Part model, mm, in its own coordinate system. Round coordinates to 2 decimals unless told otherwise and drop trailing zeros.
1) Mould opens along Y. For faces 1 (the flat face through (23132, 25, 11389)), 2 (the flat face through (23132, 0, 11389)) say: +Y half, -Y half, draft (parallel to the pull), parting line (faces both ways), or undercut.
2) Probe line 1 (Z direction, x = 23133, y = 11); line 2 (Z direction, x = 23136, y = 1.5); line 3 (X direction, y = 19.25, z = 10180.5). List the from-to ranges inside material, lowest first.
3) Drop a flat-ended pin along its axis: P1, Ø3, axis at x = 23140.5, z = 10486.5, coming from the -Y side. Give the stop position or say it passes through.
from build123d import *

# Parameters (mm, degrees)
SKETCH4_W             = 200
SKETCH4_H             = 2933.573874127
SKETCH4_R             = 12.5
BOSS_EXTRUDE1_DEPTH   = 25
SKETCH4_H_2           = 2891.000919938
BOSS_EXTRUDE1_2_DEPTH = 25
SKETCH4_H_3           = 2656.8496719
BOSS_EXTRUDE1_3_DEPTH = 25
SKETCH4_H_4           = 2167.26069873
BOSS_EXTRUDE1_4_DEPTH = 25
SKETCH4_H_5           = 1693.636583381
BOSS_EXTRUDE1_5_DEPTH = 25
SKETCH5_W             = 5252.2870397
SKETCH5_H             = 5093.660921052
CUT_EXTRUDE3_DEPTH    = 26


with BuildPart() as part:
    # Sketch4 → Boss-Extrude1 (new body)
    with BuildSketch(Plane(origin=(0, 0, 0), x_dir=(1, 0, 0), z_dir=(0, 1, 0))):
        with Locations((23132.944645813, -11409.369811035)):
            Rectangle(SKETCH4_W, SKETCH4_H)
        with Locations((23132.944645813, -12678.089615367)):
            Circle(SKETCH4_R, mode=Mode.SUBTRACT)
        with Locations((23132.944645813, -10181.030459334)):
            Circle(SKETCH4_R, mode=Mode.SUBTRACT)
    extrude(amount=BOSS_EXTRUDE1_DEPTH)


with BuildPart() as body_2:
    # Sketch4 → Boss-Extrude1 2 (new body)
    with BuildSketch(Plane(origin=(0, 0, 0), x_dir=(1, 0, 0), z_dir=(0, 1, 0))):
        with Locations((22032.944645813, -11388.083333941)):
            Rectangle(SKETCH4_W, SKETCH4_H_2)
        with Locations((22032.944645813, -12621.228285175)):
            Circle(SKETCH4_R, mode=Mode.SUBTRACT)
        with Locations((22032.944645813, -10181.030459334)):
            Circle(SKETCH4_R, mode=Mode.SUBTRACT)
    extrude(amount=BOSS_EXTRUDE1_2_DEPTH)


with BuildPart() as body_3:
    # Sketch4 → Boss-Extrude1 3 (new body)
    with BuildSketch(Plane(origin=(0, 0, 0), x_dir=(1, 0, 0), z_dir=(0, 1, 0))):
        with Locations((20832.944645813, -11271.007709922)):
            Rectangle(SKETCH4_W, SKETCH4_H_3)
        with Locations((20832.944645813, -12348.754240871)):
            Circle(SKETCH4_R, mode=Mode.SUBTRACT)
        with Locations((20832.944645813, -10181.030459334)):
            Circle(SKETCH4_R, mode=Mode.SUBTRACT)
    extrude(amount=BOSS_EXTRUDE1_3_DEPTH)


with BuildPart() as body_4:
    # Sketch4 → Boss-Extrude1 4 (new body)
    with BuildSketch(Plane(origin=(0, 0, 0), x_dir=(1, 0, 0), z_dir=(0, 1, 0))):
        with Locations((19632.944645813, -11026.213223337)):
            Rectangle(SKETCH4_W, SKETCH4_H_4)
        with Locations((19632.944645813, -11826.915448153)):
            Circle(SKETCH4_R, mode=Mode.SUBTRACT)
        with Locations((19632.944645813, -10181.030459334)):
            Circle(SKETCH4_R, mode=Mode.SUBTRACT)
    extrude(amount=BOSS_EXTRUDE1_4_DEPTH)


with BuildPart() as body_5:
    # Sketch4 → Boss-Extrude1 5 (new body)
    with BuildSketch(Plane(origin=(0, 0, 0), x_dir=(1, 0, 0), z_dir=(0, 1, 0))):
        with Locations((18802.944645813, -10789.401165663)):
            Rectangle(SKETCH4_W, SKETCH4_H_5)
        with Locations((18802.944645813, -11283.669778774)):
            Circle(SKETCH4_R, mode=Mode.SUBTRACT)
        with Locations((18802.944645813, -10181.030459334)):
            Circle(SKETCH4_R, mode=Mode.SUBTRACT)
    extrude(amount=BOSS_EXTRUDE1_5_DEPTH)


with BuildPart() as cut_extrude3_tool:
    # Sketch5 → Cut-Extrude3 (new body, through all)
    with BuildSketch(Plane(origin=(0, 0, 0), x_dir=(1, 0, 0), z_dir=(0, 1, 0))):
        with Locations((19839.936690978, -11321.244189564)):
            Rectangle(SKETCH5_W, SKETCH5_H)
    extrude(amount=CUT_EXTRUDE3_DEPTH)


with BuildPart() as body_2_1:
    add(body_2.part)

    # Cut-Extrude3: cut by cut_extrude3_tool
    add(cut_extrude3_tool.part, mode=Mode.SUBTRACT)


with BuildPart() as body_3_1:
    add(body_3.part)

    # Cut-Extrude3: cut by cut_extrude3_tool
    add(cut_extrude3_tool.part, mode=Mode.SUBTRACT)


with BuildPart() as body_4_1:
    add(body_4.part)

    # Cut-Extrude3: cut by cut_extrude3_tool
    add(cut_extrude3_tool.part, mode=Mode.SUBTRACT)


with BuildPart() as body_5_1:
    add(body_5.part)

    # Cut-Extrude3: cut by cut_extrude3_tool
    add(cut_extrude3_tool.part, mode=Mode.SUBTRACT)


solid = part.part
Reported:
1. face 1: +Y half
1. face 2: -Y half
2. line 1: z = 9942.58 to 10168.53, 10193.53 to 12665.59, 12690.59 to 12876.16
2. line 2: z = 9942.58 to 10168.91, 10193.15 to 12665.97, 12690.21 to 12876.16
2. line 3: x = 23032.94 to 23120.46, 23145.43 to 23232.94
3. P1: stops at y = 0
